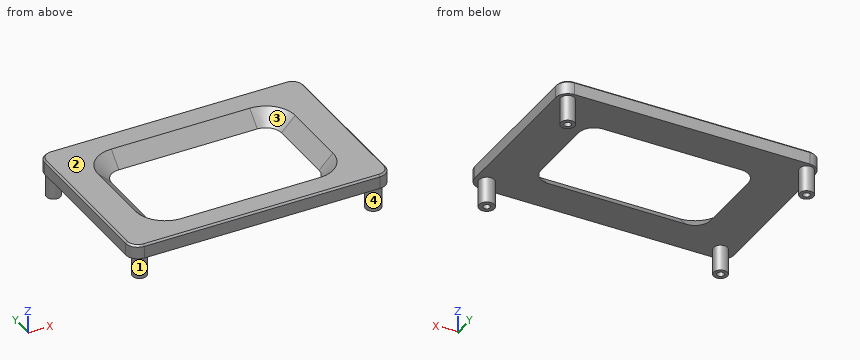
```python
from build123d import *

# Parameters (mm, degrees)
EXTRUDE_1_DEPTH     = 8
CUT_EXTRUDE_1_DEPTH = 8
CHAMFER_2_SIZE      = 1
SKETCH_3_R          = 4
SKETCH_3_R_2        = 2
EXTRUDE_3_DEPTH     = 15
SKETCH_5_R          = 4.396393258
SKETCH_5_R_2        = 2
EXTRUDE_4_DEPTH     = 15
SKETCH_9_R          = 4
SKETCH_9_R_2        = 2
EXTRUDE_5_DEPTH     = 15
SKETCH_10_R         = 4
SKETCH_10_R_2       = 2
EXTRUDE_6_DEPTH     = 15
CHAMFER_6_SIZE      = 10


with BuildPart() as part:
    # 草图1 → 凸台-拉伸1 (new body)
    with BuildSketch(Plane.XY):
        with BuildLine():
            Line((-44.320266629, 53.264700042), (91.679733371, 53.264700042))
            ThreePointArc((91.679733371, 53.264700042), (96.629480839, 51.21444751), (98.679733371, 46.264700042))
            Line((98.679733371, 46.264700042), (98.679733371, -39.735299958))
            ThreePointArc((98.679733371, -39.735299958), (96.629480839, -44.685047426), (91.679733371, -46.735299958))
            Line((91.679733371, -46.735299958), (-44.320266629, -46.735299958))
            ThreePointArc((-44.320266629, -46.735299958), (-49.270014098, -44.685047426), (-51.320266629, -39.735299958))
            Line((-51.320266629, -39.735299958), (-51.320266629, 46.264700042))
            ThreePointArc((-51.320266629, 46.264700042), (-49.270014098, 51.21444751), (-44.320266629, 53.264700042))
        make_face()
    extrude(amount=EXTRUDE_1_DEPTH)

    # 草图2 → 切除-拉伸1 (cut)
    with BuildSketch(Plane.XY.offset(8)):
        with BuildLine():
            Line((-16.295074043, 29.864928603), (63.704925957, 29.864928603))
            ThreePointArc((63.704925957, 29.864928603), (68.654673426, 27.814676072), (70.704925957, 22.864928603))
            Line((70.704925957, 22.864928603), (70.704925957, -17.135071397))
            ThreePointArc((70.704925957, -17.135071397), (68.654673426, -22.084818865), (63.704925957, -24.135071397))
            Line((63.704925957, -24.135071397), (-16.295074043, -24.135071397))
            ThreePointArc((-16.295074043, -24.135071397), (-21.244821511, -22.084818865), (-23.295074043, -17.135071397))
            Line((-23.295074043, -17.135071397), (-23.295074043, 22.864928603))
            ThreePointArc((-23.295074043, 22.864928603), (-21.244821511, 27.814676072), (-16.295074043, 29.864928603))
        make_face()
    extrude(amount=-CUT_EXTRUDE_1_DEPTH, mode=Mode.SUBTRACT)

    # 倒角2
    chamfer_2_edges = [part.edges().sort_by_distance(p)[0] for p in [
        (96.629480839, -44.685047426, 8),
        (98.679733371, 3.264700042, 8),
        (96.629480839, 51.21444751, 8),
        (23.679733371, 53.264700042, 8),
        (-49.270014098, 51.21444751, 8),
        (-51.320266629, 3.264700042, 8),
        (-49.270014098, -44.685047426, 8),
        (23.679733371, -46.735299958, 8),
    ]]
    chamfer(chamfer_2_edges, length=CHAMFER_2_SIZE)

    # 草图3 → 凸台-拉伸3 (add)
    with BuildSketch(Plane(origin=(0, 0, 0), x_dir=(-1, 0, 0), z_dir=(0, 0, -1))):
        with Locations(Location((-92.417207429, 47.443208316, 0), (0, 0, 180))):
            Circle(SKETCH_3_R)
        with Locations((-92.417207429, 47.443208316)):
            Circle(SKETCH_3_R_2, mode=Mode.SUBTRACT)
    extrude(amount=EXTRUDE_3_DEPTH)

    # 草图5 → 凸台-拉伸4 (add)
    with BuildSketch(Plane(origin=(0, 0, 0), x_dir=(-1, 0, 0), z_dir=(0, 0, -1))):
        with Locations(Location((-91.679733371, -39.735299958, 0), (0, 0, 180))):
            Circle(SKETCH_5_R)
        with Locations((-91.679733371, -39.735299958)):
            Circle(SKETCH_5_R_2, mode=Mode.SUBTRACT)
    extrude(amount=EXTRUDE_4_DEPTH)

    # 草图9 → 凸台-拉伸5 (add)
    with BuildSketch(Plane(origin=(0, 0, 0), x_dir=(-1, 0, 0), z_dir=(0, 0, -1))):
        with Locations(Location((45.596569925, 47.500240672, 0), (0, 0, 180))):
            Circle(SKETCH_9_R)
        with Locations((45.596569925, 47.500240672)):
            Circle(SKETCH_9_R_2, mode=Mode.SUBTRACT)
    extrude(amount=EXTRUDE_5_DEPTH)

    # 草图10 → 凸台-拉伸6 (add)
    with BuildSketch(Plane(origin=(0, 0, 0), x_dir=(-1, 0, 0), z_dir=(0, 0, -1))):
        with Locations(Location((42.719793233, -38.535931412, 0), (0, 0, 180))):
            Circle(SKETCH_10_R)
        with Locations((42.719793233, -38.535931412)):
            Circle(SKETCH_10_R_2, mode=Mode.SUBTRACT)
    extrude(amount=EXTRUDE_6_DEPTH)

    # 倒角6
    # the kernel refuses this chamfer: 10 mm, written as the material it takes off along each edge
    with BuildSketch(Plane(origin=(63.704925957, -24.135071397, 8), x_dir=(0, -0.9996219169112968, 0.027495876610586317), z_dir=(-1, 0, 0)), Plane(origin=(-16.295074043, 29.864928603, 8), x_dir=(0, 0.9996219169112968, 0.027495876610586317), z_dir=(1, 0, 0))) as chamfer_6_piece_1:
        Polygon((CHAMFER_6_SIZE * 0.999621916911, -CHAMFER_6_SIZE * 0.0274958766106), (-CHAMFER_6_SIZE * 0.0274958766106, -CHAMFER_6_SIZE * 0.999621916911), (0, 0), align=None)
    extrude(amount=80, mode=Mode.SUBTRACT)
    with BuildSketch(Plane(origin=(63.704925957, -17.135071397, 8), x_dir=(1, 0, 0), z_dir=(0, 1, 0))) as chamfer_6_piece_2:
        Polygon((7 + CHAMFER_6_SIZE, 0), (7, CHAMFER_6_SIZE), (7, 0), align=None)
    revolve(axis=Axis((63.704925957, -17.135071397, 8), (0, 0, -1)), revolution_arc=90, mode=Mode.SUBTRACT)
    with BuildSketch(Plane(origin=(70.704925957, 22.864928603, 8), x_dir=(0.9996219169112968, 0, 0.027495876610586317), z_dir=(0, -1, 0)), Plane(origin=(-23.295074043, -17.135071397, 8), x_dir=(-0.9996219169112968, 0, 0.02749587661058631), z_dir=(0, 1, 0))) as chamfer_6_piece_3:
        Polygon((CHAMFER_6_SIZE * 0.999621916911, -CHAMFER_6_SIZE * 0.0274958766106), (-CHAMFER_6_SIZE * 0.0274958766106, -CHAMFER_6_SIZE * 0.999621916911), (0, 0), align=None)
    extrude(amount=40, mode=Mode.SUBTRACT)
    with BuildSketch(Plane(origin=(63.704925957, 22.864928603, 8), x_dir=(0, 1, 0), z_dir=(-1, 0, 0))) as chamfer_6_piece_4:
        Polygon((7 + CHAMFER_6_SIZE, 0), (7, CHAMFER_6_SIZE), (7, 0), align=None)
    revolve(axis=Axis((63.704925957, 22.864928603, 8), (0, 0, -1)), revolution_arc=90, mode=Mode.SUBTRACT)
    with BuildSketch(Plane(origin=(-16.295074043, -17.135071397, 8), x_dir=(0, -1, 0), z_dir=(1, 0, 0))) as chamfer_6_piece_5:
        Polygon((7 + CHAMFER_6_SIZE, 0), (7, CHAMFER_6_SIZE), (7, 0), align=None)
    revolve(axis=Axis((-16.295074043, -17.135071397, 8), (0, 0, -1)), revolution_arc=90, mode=Mode.SUBTRACT)
    with BuildSketch(Plane(origin=(-16.295074043, 22.864928603, 8), x_dir=(-1, 0, 0), z_dir=(0, -1, 0))) as chamfer_6_piece_6:
        Polygon((7 + CHAMFER_6_SIZE, 0), (7, CHAMFER_6_SIZE), (7, 0), align=None)
    revolve(axis=Axis((-16.295074043, 22.864928603, 8), (0, 0, -1)), revolution_arc=90, mode=Mode.SUBTRACT)


solid = part.part
```
Work out the finished part from the listing and answer in its coordinate system (mm). Face numbers are marked on the shaded views. A direction names the side the tool comes from. Give positions to 0.01 mm unless a question says otherwise; leave off trailing zeros. Loops run counter-clockwise (first coordinate to the right, second up) from the corner with the lowest first, then second, coordinate; pieces in that order, holes last. Notation, with made-up numbers: (5.25, 32.25) -> (30.25, 32.25) arc R24 ccw to (30.25, 62.25) -> close; hole circle Ø9 at (-4.75, 88.25). An arc over 180 degrees is marked (long way). Use CSV: the item, a comma, the result in double quotes.
1. Flat-ended cylindrical pins translate along their axes: pin 1 Ø10 at (x, z) = (58.5, -5.5) entering from +Y; pin 2 Ø2 at (x, y) = (90.5, -40) entering from -Z; pin 3 Ø1.2 at (x, y) = (-42.5, -38.5) entering from -Z; pin 4 Ø1 at (x, y) = (-12, 35) entering from +Z. Find the tip coordinate at first contact, or state that the pin passes through.
Found:
pin 1,"through"
pin 2,"z = -15"
pin 3,"z = 0"
pin 4,"z = 3.64"
2. Straight lines are drawn through the part: line 1 (Y direction, x = -43.5, z = -3.75); line 2 (Z direction, x = 56, y = 44); line 3 (X direction, y = 1.5, z = 5.75). For each, find the intervals that lie inside material, in ascending order.
Found:
line 1,"-42.46 to -40.38, -36.69 to -34.61, 44.09 to 50.91"
line 2,"0 to 8"
line 3,"-51.32 to -31.05, 78.45 to 98.68"
3. The part is cut by section A-A (x = 55). Write down the section's boundary in (y, z), then the cut area to 3 significant figures.
Found:
outline,"(-46.74, 0) -> (-26.14, 0) -> (-34.14, 8) -> (-45.74, 8) -> (-46.74, 7) -> close; (31.86, 0) -> (53.26, 0) -> (53.26, 7) -> (52.26, 8) -> (39.86, 8) -> close"
area,"271 mm^2"
4. The part is cut by section C-C (z = 2.25). Write down the section's boundary in (x, y).
Found:
outline,"(-51.32, -39.74) arc R7 ccw to (-44.32, -46.74) -> (91.68, -46.74) arc R7 ccw to (98.68, -39.74) -> (98.68, 46.26) arc R7 ccw to (91.68, 53.26) -> (-44.32, 53.26) arc R7 ccw to (-51.32, 46.26) -> close; hole (-27.55, -17.14) arc R11.25 ccw to (-16.3, -28.39) -> (63.7, -28.39) arc R11.25 ccw to (74.95, -17.14) -> (74.95, 22.86) arc R11.25 ccw to (63.7, 34.11) -> (-16.3, 34.11) arc R11.25 ccw to (-27.55, 22.86) -> close"
5. A tool of negligible diameter and unlimited length cuts with its end or side. For the marked faces 3 and 4, from which of +Z, -Z, +X, -X, +Y, -Y can it reach the whole face along a straight path? Write none if from no direction.
Found:
face 3,"+Z"
face 4,"-Z"
6. The part is cut by section B-B (z = -11). Write down the section's boundary in (x, y), then the cut area to 3 significant figures.
Found:
outline,"circle Ø8 at (-45.6, 47.5); circle Ø8 at (-42.72, -38.54); circle Ø8.79 at (91.68, -39.74); circle Ø8 at (92.42, 47.44); hole circle Ø4 at (-45.6, 47.5); hole circle Ø4 at (-42.72, -38.54); hole circle Ø4 at (91.68, -39.74); hole circle Ø4 at (92.42, 47.44)"
area,"161 mm^2"
7. The mould has two halves that part along X. Classify the marked faces 1 and 2: +X half, -X half, draft (parallel to the pull), parting line (faces both ways), or undercut.
Found:
face 1,"undercut"
face 2,"draft"
